Verification items for the finished model (mm, model axes). A direction names the side the tool comes from. Coordinates: 2 decimals unless noted, no trailing zeros. Loops run counter-clockwise (first coordinate to the right, second up) from the corner with the lowest first, then second, coordinate; pieces in that order, holes last. Notation, with made-up numbers: (-6, 49.5) -> (53, 49.5) arc R19 cw to (53, 57.5) -> close; hole circle Ø3 at (23.25, 34). An arc over 180 degrees is marked (long way). Write item = value, one per line.
```python
from build123d import *

# Parameters (mm, degrees)
SKIZZE1_R                           = 0.75
AUFSATZ_LINEAR_AUSTRAGEN1_DEPTH     = 4
SCHNITT_LINEAR_START                = -3
SCHNITT_LINEAR_AUSTRAGEN2_OUTLINE_R = 0.75
SCHNITT_LINEAR_AUSTRAGEN2_DEPTH     = 3
SCHNITT_LINEAR_AUSTRAGEN3_DEPTH     = 10


# Read off the part's stored shape, not the designer's step: Schnitt-Linear austragen2
with BuildPart() as part:
    # Skizze1 → Aufsatz-Linear austragen1 (new body)
    with BuildSketch(Plane.XY):
        with BuildLine():
            ThreePointArc((-16.060120321, 8.85129891), (0, 5.725515256), (16.060120321, 8.85129891))
            ThreePointArc((16.060120321, 8.85129891), (29.189527365, 0), (16.060120321, -8.85129891))
            ThreePointArc((16.060120321, -8.85129891), (0, -5.725515256), (-16.060120321, -8.85129891))
            ThreePointArc((-16.060120321, -8.85129891), (-29.189527365, 0), (-16.060120321, 8.85129891))
        make_face()
        with Locations((-19.641235471, 0)):
            Circle(SKIZZE1_R, mode=Mode.SUBTRACT)
        with Locations((19.641235471, 0)):
            Circle(SKIZZE1_R, mode=Mode.SUBTRACT)
    extrude(amount=-AUFSATZ_LINEAR_AUSTRAGEN1_DEPTH)

    # Schnitt-Linear austragen2 outline → Schnitt-Linear austragen2 (cut)
    # profile 1 of 2: a face of its own
    with BuildSketch(Plane(origin=(0, 0, -4), x_dir=(-1, 0, 0), z_dir=(0, 0, -1)).offset(SCHNITT_LINEAR_START)):
        Polygon((20.724665483, 2.159923975), (20.316960681, 2.024603637), (20.072258051, 2.377669385), (19.719192303, 2.132966755), (19.384931733, 2.402790162), (19.115108326, 2.068529592), (18.718369619, 2.23325117), (18.553648041, 1.836512464), (18.126572608, 1.88278745), (18.080297621, 1.455712017), (17.657484574, 1.379791488), (17.733405103, 0.956978441), (17.34910824, 0.765013026), (17.541073655, 0.380716163), (17.226426423, 0.088257758), (17.518884828, -0.226389475), (17.299378073, -0.595647629), (17.668636227, -0.815154384), (17.562053082, -1.231297187), (17.978195885, -1.337880332), (17.993171082, -1.76719437), (18.42248512, -1.752219173), (18.557805458, -2.159923975), (18.965510261, -2.024603637), (19.210212891, -2.377669385), (19.563278639, -2.132966755), (19.897539209, -2.402790162), (20.167362616, -2.068529592), (20.564101323, -2.23325117), (20.728822901, -1.836512464), (21.155898334, -1.88278745), (21.20217332, -1.455712017), (21.624986367, -1.379791488), (21.549065838, -0.956978441), (21.933362701, -0.765013026), (21.741397286, -0.380716163), (22.056044519, -0.088257758), (21.763586114, 0.226389475), (21.983092869, 0.595647629), (21.613834715, 0.815154384), (21.72041786, 1.231297187), (21.304275056, 1.337880332), (21.289299859, 1.76719437), (20.859985821, 1.752219173), align=None)
        with Locations((19.641235471, 0)):
            Circle(SCHNITT_LINEAR_AUSTRAGEN2_OUTLINE_R, mode=Mode.SUBTRACT)
    # profile 2 of 2: a face of its own
    with BuildSketch(Plane(origin=(0, 0, -4), x_dir=(-1, 0, 0), z_dir=(0, 0, -1)).offset(SCHNITT_LINEAR_START)):
        Polygon((-18.557805458, 2.159923975), (-18.965510261, 2.024603637), (-19.210212891, 2.377669385), (-19.563278639, 2.132966755), (-19.897539209, 2.402790162), (-20.167362616, 2.068529592), (-20.564101323, 2.23325117), (-20.728822901, 1.836512464), (-21.155898334, 1.88278745), (-21.20217332, 1.455712017), (-21.624986367, 1.379791488), (-21.549065838, 0.956978441), (-21.933362701, 0.765013026), (-21.741397286, 0.380716163), (-22.056044519, 0.088257758), (-21.763586114, -0.226389475), (-21.983092869, -0.595647629), (-21.613834715, -0.815154384), (-21.72041786, -1.231297187), (-21.304275056, -1.337880332), (-21.289299859, -1.76719437), (-20.859985821, -1.752219173), (-20.724665483, -2.159923975), (-20.316960681, -2.024603637), (-20.072258051, -2.377669385), (-19.719192303, -2.132966755), (-19.384931733, -2.402790162), (-19.115108326, -2.068529592), (-18.718369619, -2.23325117), (-18.553648041, -1.836512464), (-18.126572608, -1.88278745), (-18.080297621, -1.455712017), (-17.657484574, -1.379791488), (-17.733405103, -0.956978441), (-17.34910824, -0.765013026), (-17.541073655, -0.380716163), (-17.226426423, -0.088257758), (-17.518884828, 0.226389475), (-17.299378073, 0.595647629), (-17.668636227, 0.815154384), (-17.562053082, 1.231297187), (-17.978195885, 1.337880332), (-17.993171082, 1.76719437), (-18.42248512, 1.752219173), align=None)
        with Locations((-19.641235471, 0)):
            Circle(SCHNITT_LINEAR_AUSTRAGEN2_OUTLINE_R, mode=Mode.SUBTRACT)
    extrude(amount=SCHNITT_LINEAR_AUSTRAGEN2_DEPTH, mode=Mode.SUBTRACT)

    # Skizze4 → Schnitt-Linear austragen3 (cut)
    with BuildSketch(Plane(origin=(0, 0, -4), x_dir=(-1, 0, 0), z_dir=(0, 0, -1))):
        with BuildLine():
            ThreePointArc((-17.558911686, -5.627070966), (-13.641235471, 0), (-17.558911686, 5.627070966))
            ThreePointArc((-17.558911686, 5.627070966), (0, 2.482397681), (17.558911686, 5.627070966))
            ThreePointArc((17.558911686, 5.627070966), (13.641235471, 0), (17.558911686, -5.627070966))
            ThreePointArc((17.558911686, -5.627070966), (0, -2.482397681), (-17.558911686, -5.627070966))
        make_face()
    extrude(amount=-SCHNITT_LINEAR_AUSTRAGEN3_DEPTH, mode=Mode.SUBTRACT)


solid = part.part
```
1) Depth check by flat-ended pin: pin 1 Ø0.9 at (x, y) = (-19.64, 0) entering from -Z; pin 2 Ø2 at (x, z) = (-9, -2.5) entering from -Y; pin 3 Ø1 at (x, z) = (-6, -2) entering from +Y; pin 4 Ø1 at (y, z) = (-2, -0.5) entering from -X. Enter the tip coordinate at first touch or a pass-through.
Ans:
pin_1 = through
pin_2 = -6.91
pin_3 = 6.22
pin_4 = -29.07
2) Release check for a two-part mould opening along Y. For faces 3 (the face through (0.23, -5.726, -1.972)), 4 (the face through (-0.23, 5.726, -1.972)), 5 (the face through (13.642, -0.102, -2.028)), 6 (the face through (0, 4, -4)) record: pulls with the +Y half, pulls with the -Y half, needs draft (parallel to the pull), parting line crosses it, or undercut.
Ans:
face_3 = pulls with the -Y half
face_4 = pulls with the +Y half
face_5 = undercut
face_6 = needs draft
3) Tool access check on faces 1 (the face through (-19, 1, -1)), 2 (the face through (29.186, 0.261, -1.972)). Record the directions out of +Z, -Z, +X, -X, +Y, -Y that give a thin tool (end or side, any length) a straight path to the whole face; none if there is none.
Ans:
face_1 = -Z
face_2 = +Z, -Z
4) Sectioned sample at B-B, the plane x = 1. Record the cut outline in (y, z), plus the area to 3 significant figures.
Ans:
outline = (-5.74, -4) -> (-2.49, -4) -> (-2.49, 0) -> (-5.74, 0) -> close; (2.49, -4) -> (5.74, -4) -> (5.74, 0) -> (2.49, 0) -> close
area = 26.0 mm2
5) Sectioned sample at C-C, the plane z = -3.1. Count the separate pieces of the cut face and the enclosed holes in it, plus the area to 3 significant figures.
Ans:
separate_pieces = 1
enclosed_holes = 3
area = 638 mm2
6) Sectioned sample at D-D, the plane x = -24. Record the cut outline in (y, z), plus the area to 3 significant figures.
Ans:
outline = (-8.5, -4) -> (8.5, -4) -> (8.5, 0) -> (-8.5, 0) -> close
area = 68.0 mm2
7) Material ranges on line 1 (X direction, y = -0.5, z = -0.5); line 2 (X direction, y = 1.5, z = -3.1); line 3 (Y direction, x = -13.5, z = -3.7), recorded low to high.
Ans:
line_1 = -29.18 to -20.2, -19.08 to -13.66, 13.66 to 19.08, 20.2 to 29.18
line_2 = -29.07 to -21.3, -18.09 to -13.83, 13.83 to 17.98, 21.2 to 29.07
line_3 = -7.91 to -4.32, 4.32 to 7.91
8) Sectioned sample at A-A, the plane y = -7.5. Record the cut outline in (x, z), plus the area to 3 significant figures.
Ans:
outline = (-25.55, -4) -> (-12.2, -4) -> (-12.2, 0) -> (-25.55, 0) -> close; (12.2, -4) -> (25.55, -4) -> (25.55, 0) -> (12.2, 0) -> close
area = 107 mm2
